The model under review builds one solid part; all positions refer to its coordinate system, in mm. Round coordinates to 2 decimals unless told otherwise and drop trailing zeros. Write each loop counter-clockwise with the first axis right and the second up, starting at its lowest first coordinate (ties: lowest second). Pieces come first, ordered by that corner, then holes. Notation, with made-up numbers: (-36.5, 20.25) - (-31.5, 20.25) arc R33 ccw to (-31.5, 52.25) - close; hole circle Ø5 at (-27.5, 76.25). An arc over 180 degrees is marked (long way). Write each question's results on one line, items separated by ' | '.
```python
from build123d import *

# Parameters (mm, degrees)
SKETCH1_R           = 31.75
BOSS_EXTRUDE1_DEPTH = 6.35
SKETCH2_R           = 3.175
SKETCH2_R_2         = 1.7
CUT_EXTRUDE1_DEPTH  = 7.35
CUT_EXTRUDE2_DEPTH  = 7.35
SKETCH4_R           = 2.2479
CUT_EXTRUDE3_DEPTH  = 7.35


with BuildPart() as part:
    # Sketch1 → Boss-Extrude1 (new body)
    with BuildSketch(Plane(origin=(0, 0, 0), x_dir=(1, 0, 0), z_dir=(0, 1, 0))):
        Circle(SKETCH1_R)
    extrude(amount=BOSS_EXTRUDE1_DEPTH)

    # Sketch2 → Cut-Extrude1 (cut, through all)
    with BuildSketch(Plane(origin=(0, 6.35, 0), x_dir=(1, 0, 0), z_dir=(0, 1, 0))):
        Circle(SKETCH2_R)
        with Locations((-5.655, 5.662415783)):
            Circle(SKETCH2_R_2)
        with Locations((5.655, 5.655)):
            Circle(SKETCH2_R_2)
        with Locations((5.655, -5.655)):
            Circle(SKETCH2_R_2)
        with Locations((-5.662415783, -5.655)):
            Circle(SKETCH2_R_2)
    extrude(amount=-CUT_EXTRUDE1_DEPTH, mode=Mode.SUBTRACT)

    # Sketch3 → Cut-Extrude2 (cut, through all)
    with BuildSketch(Plane(origin=(0, 6.35, 0), x_dir=(1, 0, 0), z_dir=(0, 1, 0))):
        with BuildLine():
            ThreePointArc((-6.96754053, 27.798227251), (-10.966989178, 26.476654013), (-14.729519838, 24.583110151))
            ThreePointArc((-14.729519838, 24.583110151), (-15.60285403, 21.098789932), (-12.118533811, 20.22545574))
            ThreePointArc((-12.118533811, 20.22545574), (-9.022957342, 21.783345987), (-5.73245947, 22.870654342))
            ThreePointArc((-5.73245947, 22.870654342), (-3.886213545, 25.951981326), (-6.96754053, 27.798227251))
        make_face()
        with BuildLine():
            ThreePointArc((-27.798227251, 6.96754053), (-26.476654013, 10.966989178), (-24.583110151, 14.729519838))
            ThreePointArc((-24.583110151, 14.729519838), (-21.098789932, 15.60285403), (-20.22545574, 12.118533811))
            ThreePointArc((-20.22545574, 12.118533811), (-21.783345987, 9.022957342), (-22.870654342, 5.73245947))
            ThreePointArc((-22.870654342, 5.73245947), (-25.951981326, 3.886213545), (-27.798227251, 6.96754053))
        make_face()
        with BuildLine():
            ThreePointArc((-27.798227251, -6.96754053), (-26.476654013, -10.966989178), (-24.583110151, -14.729519838))
            ThreePointArc((-24.583110151, -14.729519838), (-21.098789932, -15.60285403), (-20.22545574, -12.118533811))
            ThreePointArc((-20.22545574, -12.118533811), (-21.783345987, -9.022957342), (-22.870654342, -5.73245947))
            ThreePointArc((-22.870654342, -5.73245947), (-25.951981326, -3.886213545), (-27.798227251, -6.96754053))
        make_face()
        with BuildLine():
            ThreePointArc((-6.96754053, -27.798227251), (-10.966989178, -26.476654013), (-14.729519838, -24.583110151))
            ThreePointArc((-14.729519838, -24.583110151), (-15.60285403, -21.098789932), (-12.118533811, -20.22545574))
            ThreePointArc((-12.118533811, -20.22545574), (-9.022957342, -21.783345987), (-5.73245947, -22.870654342))
            ThreePointArc((-5.73245947, -22.870654342), (-3.886213545, -25.951981326), (-6.96754053, -27.798227251))
        make_face()
        with BuildLine():
            ThreePointArc((6.96754053, -27.798227251), (10.966989178, -26.476654013), (14.729519838, -24.583110151))
            ThreePointArc((14.729519838, -24.583110151), (15.60285403, -21.098789932), (12.118533811, -20.22545574))
            ThreePointArc((12.118533811, -20.22545574), (9.022957342, -21.783345987), (5.73245947, -22.870654342))
            ThreePointArc((5.73245947, -22.870654342), (3.886213545, -25.951981326), (6.96754053, -27.798227251))
        make_face()
        with BuildLine():
            ThreePointArc((27.798227251, -6.96754053), (26.476654013, -10.966989178), (24.583110151, -14.729519838))
            ThreePointArc((24.583110151, -14.729519838), (21.098789932, -15.60285403), (20.22545574, -12.118533811))
            ThreePointArc((20.22545574, -12.118533811), (21.783345987, -9.022957342), (22.870654342, -5.73245947))
            ThreePointArc((22.870654342, -5.73245947), (25.951981326, -3.886213545), (27.798227251, -6.96754053))
        make_face()
        with BuildLine():
            ThreePointArc((27.798227251, 6.96754053), (26.476654013, 10.966989178), (24.583110151, 14.729519838))
            ThreePointArc((24.583110151, 14.729519838), (21.098789932, 15.60285403), (20.22545574, 12.118533811))
            ThreePointArc((20.22545574, 12.118533811), (21.783345987, 9.022957342), (22.870654342, 5.73245947))
            ThreePointArc((22.870654342, 5.73245947), (25.951981326, 3.886213545), (27.798227251, 6.96754053))
        make_face()
        with BuildLine():
            ThreePointArc((6.96754053, 27.798227251), (10.966989178, 26.476654013), (14.729519838, 24.583110151))
            ThreePointArc((14.729519838, 24.583110151), (15.60285403, 21.098789932), (12.118533811, 20.22545574))
            ThreePointArc((12.118533811, 20.22545574), (9.022957342, 21.783345987), (5.73245947, 22.870654342))
            ThreePointArc((5.73245947, 22.870654342), (3.886213545, 25.951981326), (6.96754053, 27.798227251))
        make_face()
    extrude(amount=-CUT_EXTRUDE2_DEPTH, mode=Mode.SUBTRACT)

    # Sketch4 → Cut-Extrude3 (cut, through all)
    with BuildSketch(Plane(origin=(0, 6.35, 0), x_dir=(1, 0, 0), z_dir=(0, 1, 0))):
        with Locations((0, -25.4)):
            Circle(SKETCH4_R)
        with Locations((25.4, 0)):
            Circle(SKETCH4_R)
        with Locations((-25.4, 0)):
            Circle(SKETCH4_R)
        with Locations((0, 25.4)):
            Circle(SKETCH4_R)
    extrude(amount=-CUT_EXTRUDE3_DEPTH, mode=Mode.SUBTRACT)


solid = part.part
```
Q1. We need section A-A (x = 0). State the section outline as (y, z) points (3 decimals), plus the area to 3 significant figures.
Evaluation:
outline: (0, -31.75) - (6.35, -31.75) - (6.35, -27.648) - (0, -27.648) - close; (0, -23.152) - (6.35, -23.152) - (6.35, -3.175) - (0, -3.175) - close; (0, 3.175) - (6.35, 3.175) - (6.35, 23.152) - (0, 23.152) - close; (0, 27.648) - (6.35, 27.648) - (6.35, 31.75) - (0, 31.75) - close | area: 306 mm^2
Q2. We need section D-D (z = -9). State the section outline as (x, y) points, plus the area to 3 significant figures.
Evaluation:
outline: (-30.45, 0) - (-27.21, 0) - (-27.21, 6.35) - (-30.45, 6.35) - close; (-21.79, 0) - (21.79, 0) - (21.79, 6.35) - (-21.79, 6.35) - close; (27.21, 0) - (30.45, 0) - (30.45, 6.35) - (27.21, 6.35) - close | area: 318 mm^2
Q3. Insertion check: P1, Ø4, axis at x = 24.5, z = -15, coming from the -Y side; P2, Ø3, axis at y = 2.5, z = 14, coming from the -X side. Each pin has a flat end and moves straight along its axis. Give the tip position at first contact, or say it passes through.
Evaluation:
P1: stops at y = 0 | P2: stops at x = -29.19
Q4. The part is to be moulded in two halves that separate along X. For faces 1 (the cylindrical face through (-10.91, 3.22, -26.5)), 2 (the flat face through (0, 6.35, 7)), 3 (the cylindrical face through (-15.631, 3.219, -21.147)), say which applies: released by +X, released by -X, zero draft, split by the parting line, or undercut.
Evaluation:
face 1: undercut | face 2: zero draft | face 3: undercut
Q5. We need section C-C (z = 13). State the section outline as (x, y) points, plus the area to 3 significant figures.
Evaluation:
outline: (-28.97, 0) - (-25.54, 0) - (-25.54, 6.35) - (-28.97, 6.35) - close; (-19.9, 0) - (19.9, 0) - (19.9, 6.35) - (-19.9, 6.35) - close; (25.54, 0) - (28.97, 0) - (28.97, 6.35) - (25.54, 6.35) - close | area: 296 mm^2
Q6. For probe 1 along Z at (x, y) = (0, 5) (3 decimals); probe 2 along X at (y, z) = (1.5, 5), list the stretches that pass through material, from the lowest coordinate up.
Evaluation:
probe 1: z = -31.75 to -27.648, -23.152 to -3.175, 3.175 to 23.152, 27.648 to 31.75 | probe 2: x = -31.35 to -27.49, -23.18 to -7.23, -4.09 to 4.09, 7.22 to 23.18, 27.49 to 31.35
Q7. We need section B-B (z = 0). State the section outline as (x, y) points (3 decimals), plus the area to 3 significant figures.
Evaluation:
outline: (-31.75, 0) - (-27.648, 0) - (-27.648, 6.35) - (-31.75, 6.35) - close; (-23.152, 0) - (-3.175, 0) - (-3.175, 6.35) - (-23.152, 6.35) - close; (3.175, 0) - (23.152, 0) - (23.152, 6.35) - (3.175, 6.35) - close; (27.648, 0) - (31.75, 0) - (31.75, 6.35) - (27.648, 6.35) - close | area: 306 mm^2
